The figure shows three views and two pictorial views of one solid part (mm, origin at its lowest corner). Answer the questions. A direction names the side the tool comes from. Give positions to 0.01 mm unless a question says otherwise; leave off trailing zeros. Loops run counter-clockwise (first coordinate to the right, second up) from the corner with the lowest first, then second, coordinate; pieces in that order, holes last. Notation, with made-up numbers: M 54.5,-1 L 100.5,-1 A28 cw 100.5,35 Z; hole C 41.25,19.25 d2. An arc over 180 degrees is marked long. Answer in a Markdown table with one row per item. Add a question column.
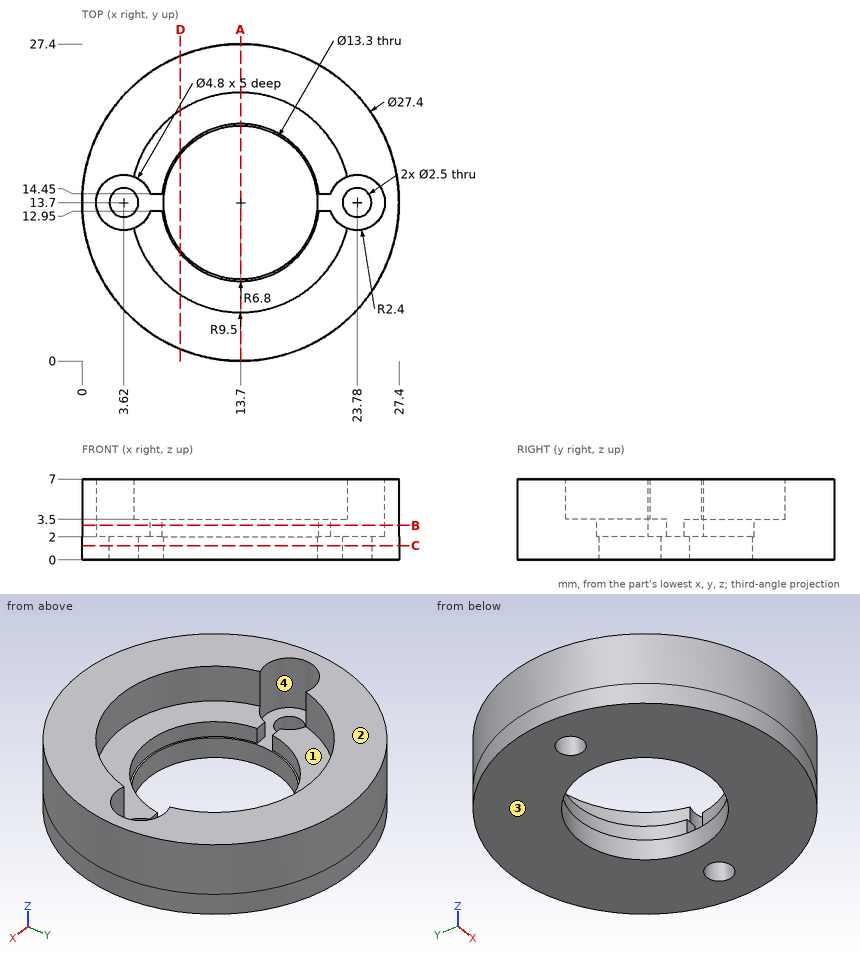
(1) The mould has two halves that part along Y. Classify the marked faces 3 and 4: pulls with the +Y half, pulls with the -Y half, needs draft (parallel to the pull), parting line crosses it, or undercut.
(2) Section D-D, the plane x = 8.5 is taken. Determine the outline of the cut face in (y, z).
(3) Which of the six approach directions +Z, -Z, +X, -X, +Y, -Y give full straight-line access (tool end or side, diameter ignored) to the marked faces 1 and 2?
(4) Section B-B, the plane z = 3 is taken. Determine the outline of the cut face in (x, y).
(5) Consider line 1 along X through (y, z) = (13.7, 3.85); line 2 along Y through (x, z) = (13.7, 1.1); line 3 along X through (y, z) = (12.75, 2.75). Determine where each line is inside the solid, lowest interval first. Write a range as from..to.
(6) Section C-C, the plane z = 1.25 is taken. Determine the outline of the cut face in (x, y).
(7) Section A-A, the plane x = 13.7 is taken. Determine the outline of the cut face in (y, z), and give its area (3 significant figures).
(8) Each of these flat-tipped pins is pushed along its axis until it touches: P1, Ø1.1, axis at x = 21, z = 3, coming from the -Y side; P2, Ø4.5, axis at x = 10, y = 10, coming from the +Z side; P3, Ø2, axis at x = 3.62, y = 13.7, coming from the +Z side; P4, Ø1.1, axis at x = 6.5, z = 2.5, coming from the -Y side. Where does it stop, or does it pass through?
Numbers:
| question | item | result |
|---|---|---|
| 1 | face 3 | needs draft |
| 1 | face 4 | undercut |
| 2 | outline | M 1.03,0 L 9.55,0 L 9.55,2 L 9.32,2 L 9.32,3.5 L 5.75,3.5 L 5.75,7 L 1.03,7 Z; M 17.85,0 L 26.37,0 L 26.37,7 L 21.65,7 L 21.65,3.5 L 18.08,3.5 L 18.08,2 L 17.85,2 Z |
| 3 | face 1 | +Z |
| 3 | face 2 | +Z, +X, -X, +Y, -Y |
| 4 | outline | C 13.7,13.7 d27.4; hole M 5.9,12.95 L 6.94,12.95 A6.8 ccw 20.46,12.95 L 21.5,12.95 A2.4 ccw long 21.5,14.45 L 20.46,14.45 A6.8 ccw 6.94,14.45 L 5.9,14.45 A2.4 ccw long Z |
| 5 | line 1 | x = 0..1.22, 26.18..27.4 |
| 5 | line 2 | y = 0..7.05, 20.35..27.4 |
| 5 | line 3 | x = 0.03..1.42, 5.82..6.97, 20.43..21.58, 25.98..27.37 |
| 6 | outline | C 13.7,13.7 d27.4; hole C 3.62,13.7 d2.5; hole C 13.7,13.7 d13.3; hole C 23.78,13.7 d2.5 |
| 7 | outline | M 0,0 L 7.05,0 L 7.05,2 L 6.9,2 L 6.9,3.5 L 4.2,3.5 L 4.2,7 L 0,7 Z; M 20.35,0 L 27.4,0 L 27.4,7 L 23.2,7 L 23.2,3.5 L 20.5,3.5 L 20.5,2 L 20.35,2 Z |
| 7 | area | 78.3 mm² |
| 8 | P1 | stops at y = 1.78 |
| 8 | P2 | stops at z = 3.5 |
| 8 | P3 | passes through |
| 8 | P4 | stops at y = 1.72 |
